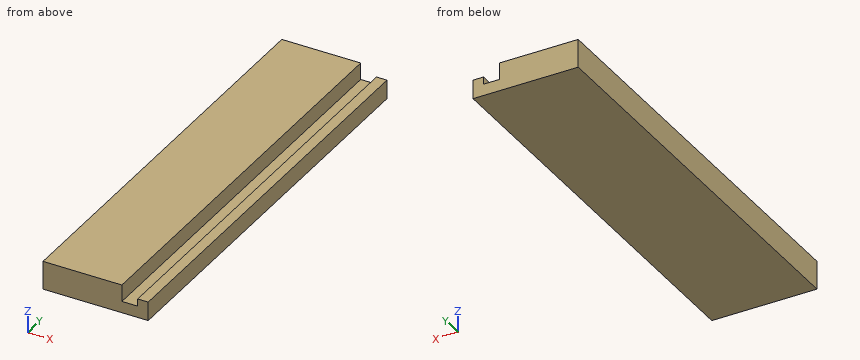
```python
from build123d import *

# Parameters (mm, degrees)
F2_DEPTH = 27
F1_W     = 15
F1_H     = 400
F3_DEPTH = 11
F1_W_2   = 10
F4_DEPTH = 18


# Not quite as in the source:
# - a feature of the source that left no trace in its solid (it failed there, or was rolled back) is left out


with BuildPart() as f2:
    # F1 (on Top) → F2 (new body)
    with BuildSketch(Plane.XY):
        with BuildLine():
            Line((-1.25, 200), (-37.5, 200))
            Line((-37.5, 200), (-37.5, -200))
            Line((-37.5, -200), (37.5, -200))
            Line((37.5, -200), (37.5, 200))
            Line((37.5, 200), (1.25, 200))
            Line((1.25, 200), (1.25, -184.1316527028))
            ThreePointArc((1.25, -184.1316527028), (4.6636895265, -186.2250827824), (6, -190))
            ThreePointArc((6, -190), (-3.7749172176, -194.6636895265), (-1.25, -184.1316527028))
            Line((-1.25, -184.1316527028), (-1.25, 200))
        make_face()
        with BuildLine():
            Line((1.25, 200), (-1.25, 200))
            Line((-1.25, 200), (-1.25, -184.1316527028))
            ThreePointArc((-1.25, -184.1316527028), (0, -184), (1.25, -184.1316527028))
            Line((1.25, -184.1316527028), (1.25, 200))
        make_face()
        with BuildLine():
            ThreePointArc((1.25, -184.1316527028), (0, -184), (-1.25, -184.1316527028))
            ThreePointArc((-1.25, -184.1316527028), (-3.7749172176, -194.6636895265), (6, -190))
            ThreePointArc((6, -190), (4.6636895265, -186.2250827824), (1.25, -184.1316527028))
        make_face()
    extrude(amount=F2_DEPTH)

    # F1 (on Top) → F3 (join)
    with BuildSketch(Plane.XY):
        with Locations((45, 0)):
            Rectangle(F1_W, F1_H)
    extrude(amount=F3_DEPTH)

    # F1 (on Top) → F4 (join)
    with BuildSketch(Plane.XY):
        with Locations((57.5, 0)):
            Rectangle(F1_W_2, F1_H)
    extrude(amount=F4_DEPTH)


solid = f2.part
```
For this review, take the finished solid that the model builds, in its own axes (mm). Round coordinates to 2 decimals unless told otherwise and drop trailing zeros. Write each loop counter-clockwise with the first axis right and the second up, starting at its lowest first coordinate (ties: lowest second). Pieces come first, ordered by that corner, then holes. Notation, with made-up numbers: (61, 43) -> (99, 43) arc R29 ccw to (99, 67) -> close; hole circle Ø2 at (66.25, -39). An arc over 180 degrees is marked (long way). One line per question, with ' | ' between items. Start each with the question number.
1) Wall thickness on line 1 along X through (y, z) = (-31.5, 17.75); line 2 along Z through (x, y) = (50, 116.5); line 3 along X through (y, z) = (-56.5, 23.5): over which ranges is each line inside the solid? List them lowest first.
2) For pin 1 Ø4.5 at (x, y) = (47, 82.5) entering from +Z; pin 2 Ø8 at (x, y) = (59, 80) entering from +Z, all flat-tipped, find the tip position at first contact; note any pin that passes through.
3) Add section C-C (z = 22.75). Write out the cut boundary in (x, y), and give its area (3 significant figures).
4) Add section B-B (x = 45). Write out the cut boundary in (y, z), and give its area (3 significant figures).
5) Add section A-A (y = 86). Write out the cut boundary in (x, z), and give its area (3 significant figures).
Reported:
1) line 1: x = -37.5 to 37.5, 52.5 to 62.5 | line 2: z = 0 to 11 | line 3: x = -37.5 to 37.5
2) pin 1: stops at z = 11 | pin 2: stops at z = 18
3) outline: (-37.5, -200) -> (37.5, -200) -> (37.5, 200) -> (-37.5, 200) -> close | area: 30,000 mm²
4) outline: (-200, 0) -> (200, 0) -> (200, 11) -> (-200, 11) -> close | area: 4,400 mm²
5) outline: (-37.5, 0) -> (62.5, 0) -> (62.5, 18) -> (52.5, 18) -> (52.5, 11) -> (37.5, 11) -> (37.5, 27) -> (-37.5, 27) -> close | area: 2,370 mm²
